Geometry check sheet. Reference: the model listing, model coordinates, mm. A direction names the side the tool comes from. Round coordinates to 2 decimals unless told otherwise and drop trailing zeros. Loops run counter-clockwise (first coordinate to the right, second up) from the corner with the lowest first, then second, coordinate; pieces in that order, holes last. Notation, with made-up numbers: M 55.5,-1 L 90.5,-1 A11 ccw 90.5,3 Z; hole C -3,86.5 d8. An arc over 180 degrees is marked long. Use one line per item in the form item = value. Start each with the question number.
1. Go/stop test with flat-tipped pins: pin 1 (1.5 mm diameter, centred on y = 10.5, z = -25.5, fed in from +X); pin 2 (2 mm diameter, centred on y = -4, z = -29, fed in from -X); pin 3 (5 mm diameter, centred on y = -5, z = -5, fed in from +X) (3 decimals). Record where each tip stops, or that it passes through.
2. Cross-section at B-B (y = 0). Record the boundary of the cut face in (x, z).
3. Cross-section at D-D (z = -14). Record the boundary of the cut face in (x, y), then the cut area to 3 significant figures.
4. Material ranges on line 1 (Y direction, x = 0, z = -27.5); line 2 (Z direction, x = -9.5, y = -9.25); line 3 (Z direction, x = 1.75, y = -5.25), recorded low to high.
5. Cross-section at C-C (x = 0). Record the boundary of the cut face in (y, z), then the cut area to 3 significant figures.
6. Cross-section at A-A (x = -11). Record the boundary of the cut face in (y, z), then the cut area to 3 significant figures.
7. Set-up check for faces 5 (the flat face through (0, 0, -39)), 6 (the flat face through (0, 0, -45)), 7 (the cylindrical face through (-4.917, -12.335, -22.21)): record each of +Z, -Z, +X, -X, +Y, -Y from which the full face is reachable in a straight line by a thin tool's end or side.
8. Draft check along X on faces 1 (the cylindrical face through (13.35, -4.21, -22.18)), 2 (the cylindrical face through (-4.88, 12.33, -22.21)), 3 (the cylindrical face through (12.498, -0.55, -23.224)), 4 (the flat face through (0, 0, 0)). Enter one of: pulls with the +X half, pulls with the -X half, needs draft (parallel to the pull), parting line crosses it, or undercut.
```python
from build123d import *

# Parameters (mm, degrees)
CYLINDER003_R     = 12.51
CYLINDER003_DEPTH = 30
CYLINDER002_R     = 12.51
CYLINDER002_DEPTH = 32
CYLINDER001_R     = 14
CYLINDER001_DEPTH = 45


with BuildPart() as cylinder003:
    # Cylinder003 → Cylinder003 (new body)
    with BuildSketch(Plane(origin=(-7, 0, -37), x_dir=(-1, 0, 0), z_dir=(0, 0, 1))):
        Circle(CYLINDER003_R)
    extrude(amount=CYLINDER003_DEPTH)


with BuildPart() as cylinder002:
    # Cylinder002 → Cylinder002 (new body)
    with BuildSketch(Plane(origin=(0, 0, -39), x_dir=(-1, 0, 0), z_dir=(0, 0, 1))):
        Circle(CYLINDER002_R)
    extrude(amount=CYLINDER002_DEPTH)


with BuildPart() as cut001:
    # Cylinder001 → Cylinder001 (new body)
    with BuildSketch(Plane(origin=(0, 0, 0), x_dir=(1, 0, 0), z_dir=(0, 0, -1))):
        Circle(CYLINDER001_R)
    extrude(amount=CYLINDER001_DEPTH)

    # Cut: cut Cylinder002
    add(cylinder002.part, mode=Mode.SUBTRACT)

    # Cut001: cut Cylinder003
    add(cylinder003.part, mode=Mode.SUBTRACT)


solid = cut001.part
```
Reported:
q1.pin_1 = 10.05
q1.pin_2 = 11.47
q1.pin_3 = 13.775
q2.outline = M -14,-45 L 14,-45 L 14,0 L -14,0 L -14,-7 L 12.51,-7 L 12.51,-39 L -12.51,-39 L -12.51,-37 L -14,-37 Z
q3.outline = M -6.32,-12.49 A14 ccw long -6.32,12.49 A12.51 cw -3.5,12.01 A12.51 cw long -3.5,-12.01 A12.51 cw Z
q3.area = 77.0 mm²
q4.line_1 = -14 to -12.51, 12.51 to 14
q4.line_2 = -45 to -37, -7 to 0
q4.line_3 = -45 to -39, -7 to 0
q5.outline = M -14,-45 L 14,-45 L 14,0 L -14,0 Z; hole M -12.51,-39 L 12.51,-39 L 12.51,-7 L -12.51,-7 Z
q5.area = 459 mm²
q6.outline = M -8.66,-45 L 8.66,-45 L 8.66,-37 L 5.96,-37 L 5.96,-39 L -5.96,-39 L -5.96,-37 L -8.66,-37 Z; M -8.66,-7 L 8.66,-7 L 8.66,0 L -8.66,0 Z
q6.area = 236 mm²
q7.face_5 = none
q7.face_6 = -Z, +X, -X, +Y, -Y
q7.face_7 = -X
q8.face_1 = parting line crosses it
q8.face_2 = pulls with the -X half
q8.face_3 = undercut
q8.face_4 = needs draft
